Verification items for the finished model (mm, model axes). Face numbers are marked on the shaded views. A direction names the side the tool comes from. Give positions to 0.01 mm unless a question says otherwise; leave off trailing zeros. Write each loop counter-clockwise with the first axis right and the second up, starting at its lowest first coordinate (ties: lowest second). Pieces come first, ordered by that corner, then holes. Notation, with made-up numbers: (70, 25) -> (105, 25) arc R25 cw to (105, 58) -> close; hole circle Ø5 at (4, 35.25). An arc over 180 degrees is marked (long way). Use CSV: the item, a comma, the result in double quotes. Start each with the question number.
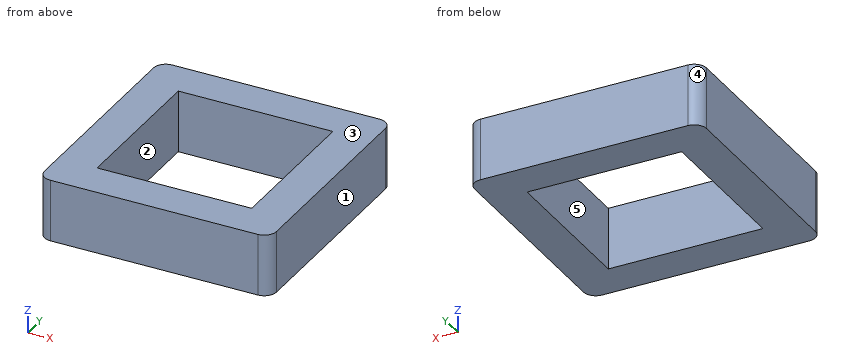
Autodesk Inventor part; units mm, degrees
ref_plane "YZ Plane" through (0, 0, 0) normal (1, 0, 0) x (0, 1, 0)
ref_plane "XZ Plane" through (0, 0, 0) normal (0, 1, 0) x (-1, 0, 0)
ref_plane "XY Plane" through (0, 0, 0) normal (0, 0, 1) x (1, 0, 0)
sketch "Sketch1" plane through (0, 0, 0) normal (0, 0, 1) x (1, 0, 0)
  line L0 (-30, -30) -> (30, -30)
  line L1 (30, -30) -> (30, 30)
  line L2 (30, 30) -> (-30, 30)
  line L3 (-30, 30) -> (-30, -30)
  line L4 (-30, -30) -> (30, 30) construction
  line L5 (30, -30) -> (-30, 30) construction
  point P0 (0, 0)
  dimension "d0" = 60
extrude "Extrusion1" add sketch "Sketch1" against normal blind 16
fillet "Fillet1" radius 3.175 4 edges at (-30, 30, -8) (30, 30, -8) (30, -30, -8) (-30, -30, -8)
sketch "Sketch2" plane through (0, 0, 0) normal (0, 0, 1) x (1, 0, 0)
  line L0 (-20, -20) -> (20, -20)
  line L1 (20, -20) -> (20, 20)
  line L2 (20, 20) -> (-20, 20)
  line L3 (-20, 20) -> (-20, -20)
  line L4 (-20, -20) -> (20, 20) construction
  line L5 (20, -20) -> (-20, 20) construction
  point P0 (0, 0)
  dimension "d4" = 40
extrude "Extrusion2" cut sketch "Sketch2" against normal blind 16
properties part number "Fan 60x60x16"
(1) Draft check along Y on the marked faces 3, 4 and 5. Enter one of: released by +Y, released by -Y, zero draft, split by the parting line, or undercut.
(2) Section check C-C on z = -9. Record the cut outline in (x, y) (3 decimals).
(3) Section check A-A on y = -5. Record the cut outline in (x, z), then the cut area to 3 significant figures.
(4) Set-up check for the marked faces 1 and 2: record each of +Z, -Z, +X, -X, +Y, -Y from which the full face is reachable in a straight line by a thin tool's end or side.
(5) Thickness scan on line 1 (X direction, y = 12, z = -1.75). Record the ranges inside material, lowest first. Write a range as from..to.
Data:
1,face 3,"zero draft"
1,face 4,"released by +Y"
1,face 5,"undercut"
2,outline,"(-30, -26.825) arc R3.175 ccw to (-26.825, -30) -> (26.825, -30) arc R3.175 ccw to (30, -26.825) -> (30, 26.825) arc R3.175 ccw to (26.825, 30) -> (-26.825, 30) arc R3.175 ccw to (-30, 26.825) -> close; hole (-20, -20) -> (20, -20) -> (20, 20) -> (-20, 20) -> close"
3,outline,"(-30, -16) -> (-20, -16) -> (-20, 0) -> (-30, 0) -> close; (20, -16) -> (30, -16) -> (30, 0) -> (20, 0) -> close"
3,area,"320 mm2"
4,face 1,"+Z, -Z, +X, +Y, -Y"
4,face 2,"+Z, -Z"
5,line 1,"x = -30..-20, 20..30"
